Autodesk Inventor part; units mm, degrees
ref_plane "YZ Plane" through (0, 0, 0) normal (1, 0, 0) x (0, 1, 0)
ref_plane "XZ Plane" through (0, 0, 0) normal (0, 1, 0) x (-1, 0, 0)
ref_plane "XY Plane" through (0, 0, 0) normal (0, 0, 1) x (1, 0, 0)
sketch "Sketch1" plane through (0, 0, 0) normal (0, 1, 0) x (-1, 0, 0)
  circle A0 centre (0, 0) radius 14.15
  circle A1 centre (0, 0) radius 12.1
  dimension "d3" = 28.3
  dimension "d6" = 24.2
extrude "Extrusion1" add sketch "Sketch1" along normal blind 40 contours A0 | A1
sketch "Sketch3" plane through (0, 0, 0) normal (0, -1, 0) x (1, 0, 0)
  circle A0 centre (0, 0) radius 12.1
  dimension "d10" = 24.2
extrude "Extrusion3" cut sketch "Sketch3" against normal blind 40
sketch "Sketch4" plane through (0, 0, 0) normal (0, -1, 0) x (1, 0, 0)
  circle A0 centre (0, 0) radius 13
  dimension "d13" = 26
extrude "Extrusion4" cut sketch "Sketch4" against normal blind 20
properties part number "_3DPrint"
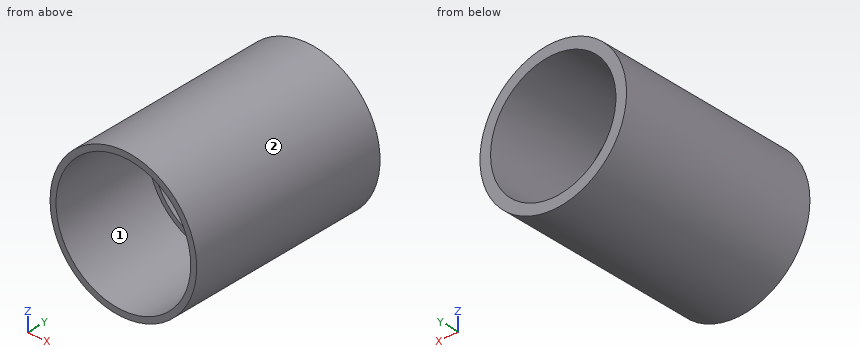
Geometry check sheet. Reference: the model listing, model coordinates, mm. Face numbers are marked on the shaded views. Round coordinates to 2 decimals unless told otherwise and drop trailing zeros. Write each loop counter-clockwise with the first axis right and the second up, starting at its lowest first coordinate (ties: lowest second). Pieces come first, ordered by that corner, then holes. Notation, with made-up numbers: (20, 16) -> (30, 16) arc R25 cw to (30, 55) -> close; hole circle Ø5 at (30, -19). An arc over 180 degrees is marked (long way). One line per item, written item: value. Start each with the question number.
(1) Cross-section at D-D, the plane y = 9. Record the cut outline in (x, z), and give its area (3 significant figures).
(2) Go/stop test with flat-tipped pins: pin 1 Ø1 at (y, z) = (23.5, 2) entering from +X; pin 2 Ø2 at (x, z) = (8.5, 3.5) entering from -Y; pin 3 Ø1.5 at (x, y) = (-11, 17) entering from -Z (3 decimals); pin 4 Ø3 at (y, z) = (28.5, -9) entering from -X. Record where each tip stops, or that it passes through.
(3) Cross-section at B-B, the plane z = 0. Record the cut outline in (x, y), and give its area (3 significant figures).
(4) Draft check along Z on the marked faces 1 and 2. Enter one of: +Z half, -Z half, draft (parallel to the pull), parting line (faces both ways), or undercut.
(5) Cross-section at A-A, the plane x = 0. Record the cut outline in (y, z), and give its area (3 significant figures).
(6) Scan lines: line 1 (Z direction, x = 0, y = 14.25); line 2 (Z direction, x = 0, y = 26); line 3 (X direction, y = 22, z = -8). Record each from-to range of solid material in increasing order. Write a range as [from, to].
(7) Cross-section at C-C, the plane y = 25. Record the cut outline in (x, z).
Answer:
1. outline: circle Ø28.3 at (0, 0); hole circle Ø26 at (0, 0)
1. area: 98.1 mm²
2. pin 1: x = 14.07
2. pin 2: through
2. pin 3: z = -9.755
2. pin 4: x = -12
3. outline: (-14.15, 0) -> (-13, 0) -> (-13, 20) -> (-12.1, 20) -> (-12.1, 40) -> (-14.15, 40) -> close; (12.1, 20) -> (13, 20) -> (13, 0) -> (14.15, 0) -> (14.15, 40) -> (12.1, 40) -> close
3. area: 128 mm²
4. face 1: undercut
4. face 2: parting line
5. outline: (0, -14.15) -> (40, -14.15) -> (40, -12.1) -> (20, -12.1) -> (20, -13) -> (0, -13) -> close; (0, 13) -> (20, 13) -> (20, 12.1) -> (40, 12.1) -> (40, 14.15) -> (0, 14.15) -> close
5. area: 128 mm²
6. line 1: [-14.15, -13], [13, 14.15]
6. line 2: [-14.15, -12.1], [12.1, 14.15]
6. line 3: [-11.67, -9.08], [9.08, 11.67]
7. outline: circle Ø28.3 at (0, 0); hole circle Ø24.2 at (0, 0)
